Input: part model. Units: mm. Frame: model coordinates. Face numbers are marked on the shaded views. A direction names the side the tool comes from. Coordinates: 2 decimals unless noted, no trailing zeros. Write each loop counter-clockwise with the first axis right and the second up, starting at its lowest first coordinate (ties: lowest second). Pieces come first, ordered by that corner, then holes. Notation, with made-up numbers: M 30,9.5 L 62,9.5 A33 ccw 62,46.5 Z; hole C 14.5,-19.5 d11. An arc over 180 degrees is marked long. Answer as a JSON object with one key per item and string values. Group by question number.
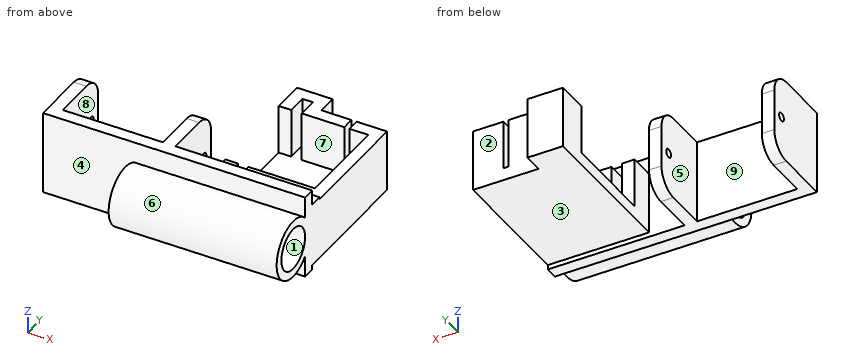
from build123d import *

# Parameters (mm, degrees)
SKETCH1_W           = 50
SKETCH1_H           = 20
BOSS_EXTRUDE1_DEPTH = 3
SKETCH2_W           = 3
SKETCH2_H           = 20
BOSS_EXTRUDE2_DEPTH = 15
SKETCH3_R           = 1
CUT_EXTRUDE1_DEPTH  = 15
FILLET1_R           = 5
SKETCH4_W           = 3
SKETCH4_H           = 20
BOSS_EXTRUDE3_DEPTH = 15
CUT_EXTRUDE2_START  = -15
SKETCH5_R           = 1
CUT_EXTRUDE2_DEPTH  = 15
FILLET2_R           = 5
BOSS_EXTRUDE4_DEPTH = 5.9
SKETCH7_W           = 20
SKETCH7_H           = 3
BOSS_EXTRUDE5_DEPTH = 12.8
SKETCH8_W           = 15.8
SKETCH8_H           = 3.1
BOSS_EXTRUDE6_DEPTH = 6.4
BOSS_EXTRUDE7_DEPTH = 3
SKETCH10_W          = 43.689261584
SKETCH10_H          = 59.678024431
CUT_EXTRUDE4_DEPTH  = 0.2
SKETCH11_R          = 7
SKETCH11_R_2        = 5
BOSS_EXTRUDE8_DEPTH = 40.2


with BuildPart() as part:
    # Sketch1 → Boss-Extrude1 (new body)
    with BuildSketch(Plane(origin=(0, 0, 0), x_dir=(1, 0, 0), z_dir=(0, 1, 0))):
        with Locations((25, -10)):
            Rectangle(SKETCH1_W, SKETCH1_H)
    extrude(amount=BOSS_EXTRUDE1_DEPTH)

    # Sketch2 → Boss-Extrude2 (add)
    with BuildSketch(Plane(origin=(0, 3, 0), x_dir=(1, 0, 0), z_dir=(0, 1, 0))):
        with Locations((1.5, -10)):
            Rectangle(SKETCH2_W, SKETCH2_H)
    extrude(amount=BOSS_EXTRUDE2_DEPTH)

    # Sketch3 → Cut-Extrude1 (cut)
    with BuildSketch(Plane(origin=(3, 0, 0), x_dir=(0, 0, -1), z_dir=(1, 0, 0))):
        with Locations((-10, 15)):
            Circle(SKETCH3_R)
    extrude(amount=-CUT_EXTRUDE1_DEPTH, mode=Mode.SUBTRACT)

    # Fillet1
    fillet1_edges = [part.edges().sort_by_distance(p)[0] for p in [
        (1.5, 18, 20),
        (1.5, 18, 0),
    ]]
    fillet(fillet1_edges, radius=FILLET1_R)

    # Sketch4 → Boss-Extrude3 (add)
    with BuildSketch(Plane(origin=(0, 3, 0), x_dir=(1, 0, 0), z_dir=(0, 1, 0))):
        with Locations((28.5, -10)):
            Rectangle(SKETCH4_W, SKETCH4_H)
    extrude(amount=BOSS_EXTRUDE3_DEPTH)

    # Sketch5 → Cut-Extrude2 (cut)
    with BuildSketch(Plane.ZY.offset(-27).offset(CUT_EXTRUDE2_START)):
        with Locations(Location((10, 15, 0), (0, 0, 180))):
            Circle(SKETCH5_R)
    extrude(amount=CUT_EXTRUDE2_DEPTH, mode=Mode.SUBTRACT)

    # Fillet2
    fillet2_edges = [part.edges().sort_by_distance(p)[0] for p in [
        (28.5, 18, 20),
        (28.5, 18, 0),
    ]]
    fillet(fillet2_edges, radius=FILLET2_R)

    # Sketch6 → Boss-Extrude4 (add, symmetric)
    with BuildSketch(Plane(origin=(0, 0, 10), x_dir=(-1, 0, 0), z_dir=(0, 0, -1))):
        Polygon((-38.5, 31.6), (-38.5, 34.6), (-38.5, 39.3), (-47, 39.3), (-47, 34.6), (-54.2, 34.6), (-54.2, 31.6), (-44, 31.6), (-44, 36.3), (-41.5, 36.3), (-41.5, 31.6), align=None)
        Polygon((-38.5, 1.4), (-38.5, 6.1), (-38.5, 9.1), (-41.5, 9.1), (-41.5, 4.4), (-44, 4.4), (-44, 9.1), (-59.9, 9.1), (-59.9, 31.6), (-55.4, 31.6), (-55.4, 34.6), (-62.9, 34.6), (-62.9, 6.1), (-47, 6.1), (-47, 1.4), align=None)
    extrude(amount=BOSS_EXTRUDE4_DEPTH, both=True)


with BuildPart() as boss_extrude4_piece_1:
    # of the separate pieces the step leaves, piece 1, a body of its own (boss_extrude4_pieces)
    add(part.part.solids().sort_by_distance((27, 13, 0))[0])

    # Sketch7 → Boss-Extrude5 (add)
    with BuildSketch(Plane(origin=(50, 0, 0), x_dir=(0, 0, -1), z_dir=(1, 0, 0))):
        with Locations((-10, 1.5)):
            Rectangle(SKETCH7_W, SKETCH7_H)
    extrude(amount=BOSS_EXTRUDE5_DEPTH)

    # Sketch8 → Boss-Extrude6 (add, symmetric)
    with BuildSketch(Plane(origin=(0, 0, 10), x_dir=(-1, 0, 0), z_dir=(0, 0, -1))):
        with Locations((-54.9, 4.55)):
            Rectangle(SKETCH8_W, SKETCH8_H)
    extrude(amount=BOSS_EXTRUDE6_DEPTH, both=True)



with BuildPart() as boss_extrude4_piece_2:
    # of the separate pieces the step leaves, piece 2, a body of its own (boss_extrude4_pieces)
    add(part.part.solids().sort_by_distance((38.5, 31.6, 15.9))[0])


with BuildPart() as boss_extrude4_piece_1_1:
    add(boss_extrude4_piece_1.part)

    add(boss_extrude4_piece_2.part)  # Boss-Extrude7 merges Boss-Extrude4 piece 2
    # Sketch9 → Boss-Extrude7 (add)
    with BuildSketch(Plane(origin=(0, 0, 4.1), x_dir=(-1, 0, 0), z_dir=(0, 0, -1))):
        Polygon((-38.5, 3), (-38.5, 39.3), (-47, 39.3), (-47, 34.6), (-62.9, 34.6), (-62.8, 3), align=None)
    extrude(amount=BOSS_EXTRUDE7_DEPTH)

    # Sketch10 → Cut-Extrude4 (cut)
    with BuildSketch(Plane(origin=(62.9, 0, 0), x_dir=(0, 0, -1), z_dir=(1, 0, 0))):
        with Locations((-9.388309177, 18.772485295)):
            Rectangle(SKETCH10_W, SKETCH10_H)
    extrude(amount=-CUT_EXTRUDE4_DEPTH, mode=Mode.SUBTRACT)

    # Sketch11 → Boss-Extrude8 (add)
    with BuildSketch(Plane(origin=(62.7, 0, 0), x_dir=(0, 0, -1), z_dir=(1, 0, 0))):
        with Locations((-10, -5)):
            Circle(SKETCH11_R)
        with Locations((-10, -5)):
            Circle(SKETCH11_R_2, mode=Mode.SUBTRACT)
    extrude(amount=-BOSS_EXTRUDE8_DEPTH)


solid = boss_extrude4_piece_1_1.part
Q1. Access query for the marked faces 1, 2, 3, 4 and 5. Directions: +Z, -Z, +X, -X, +Y, -Y. A direction counts if a zero-diameter tool reaches every point of the face in a straight line with its end or side. Return the directions, or none.
Q2. Section B-B, the plane x = 36. Return the cut outline in (y, z), and give its area (3 significant figures).
Q3. Section D-D, the plane z = 18.5. Return the cut outline in (x, y), and give its area (3 significant figures).
Q4. Draft query along Y for the marked faces 6, 7, 8 and 9. Return one class per face: released by +Y, released by -Y, zero draft, split by the parting line, or undercut.
Q5. Section C-C, the plane y = 11.5. Return the cut outline in (x, z), and give its area (3 significant figures).
Q6. Line query: line 1 (X direction, y = 7.5, z = 13.25); line 2 (X direction, y = 13, z = 11.25); line 3 (X direction, y = 36, z = 12). Output: solid intervals per line, ascending. Write a range as from..to.
Q7. Section A-A, the plane y = -5. Return the cut outline in (x, z).
Q8. Pin query (flat end, axial travel): pin 1 Ø3 at (x, z) = (49.5, 9.5) entering from +Y; pin 2 Ø4 at (y, z) = (34, 8.5) entering from -X; pin 3 Ø1.5 at (x, z) = (1.5, 10.5) entering from +Y; pin 4 Ø10 at (y, z) = (18, 10.5) entering from -X. Return the tip coordinate at first contact, or that it passes through.
Filled in:
{
 "1": {"face 1": "+X, -X", "face 2": "+Z, -Z, +X, +Y", "face 3": "-Z, +X, +Y", "face 4": "-X", "face 5": "+Z, -Z, +Y"},
 "2": {"outline": "M 0,0 L 3,0 L 3,20 L 0,20 L 0,14.9 A7 ccw long 0,5.1 Z; hole C -5,10 d10", "area": "122 mm^2"},
 "3": {"outline": "M 0,0 L 62.7,0 L 62.7,3 L 30,3 L 30,16.57 L 27,16.57 L 27,3 L 3,3 L 3,16.57 L 0,16.57 Z", "area": "270 mm^2"},
 "4": {"face 6": "undercut", "face 7": "undercut", "face 8": "zero draft", "face 9": "released by +Y"},
 "5": {"outline": "M 0,0 L 3,0 L 3,20 L 0,20 Z; M 27,0 L 30,0 L 30,20 L 27,20 Z; M 38.5,1.1 L 62.7,1.1 L 62.7,15.9 L 59.9,15.9 L 59.9,4.1 L 38.5,4.1 Z", "area": "226 mm^2"},
 "6": {"line 1": "0..3, 27..30, 38.5..41.5, 44..62.7", "line 2": "0..3, 27..30, 59.9..62.7", "line 3": "38.5..41.5, 44..47"},
 "7": {"outline": "M 22.5,3 L 62.7,3 L 62.7,5 L 22.5,5 Z; M 22.5,15 L 62.7,15 L 62.7,17 L 22.5,17 Z"},
 "8": {"pin 1": "y = 34.6", "pin 2": "x = 38.5", "pin 3": "y = 18", "pin 4": "x = 0"}
}
